```python
from build123d import *

# Parameters (mm, degrees)
SKETCH1_R               = 10
BOSS_EXTRUDE1_DEPTH     = 2
CUT_EXTRUDE1_REACH      = 16.283
CUT_EXTRUDE1_END_RADIUS = 10
SKETCH2_R               = 1.5
CUT_EXTRUDE1_DRAFT      = 2
CIRPATTERN1_COUNT       = 3


with BuildPart() as part:
    # Sketch1 → Boss-Extrude1 (new, symmetric)
    with BuildSketch(Plane(origin=(0, 0, 0), x_dir=(1, 0, 0), z_dir=(0, 1, 0))):
        with Locations(Location((0, 0, 0), (0, 0, 270))):
            Circle(SKETCH1_R)
        Polygon((0, 3.868246804), (-3.35, 1.934123402), (-3.35, -1.934123402), (0, -3.868246804), (3.35, -1.934123402), (3.35, 1.934123402), align=None, mode=Mode.SUBTRACT)
    extrude(amount=BOSS_EXTRUDE1_DEPTH, both=True)

    # Cut-Extrude1: up to this cylinder (the profile starts inside it)
    cut_extrude1_end = Plane(origin=(0, 0, 0), z_dir=(0, -1, 0)) * Cylinder(CUT_EXTRUDE1_END_RADIUS, 53.566, mode=Mode.PRIVATE)



with BuildPart() as cut_extrude1_long_prism_1:
    # Sketch2 → Cut-Extrude1 (the long prism of profile 1, to be tilted and cut off)
    with BuildSketch(Plane.XY):
        Circle(SKETCH2_R)
    extrude(amount=CUT_EXTRUDE1_REACH)
    cut_extrude1_tool1_sides = [cut_extrude1_long_prism_1.faces().sort_by_distance(p)[0] for p in [
        (-1.5, 0, 8.1415),
    ]]
    draft(cut_extrude1_tool1_sides, Plane.XY, CUT_EXTRUDE1_DRAFT)  # the draft: side faces tilted about the start plane


with BuildPart() as part_1:
    add(part.part)
    cut_extrude1_tool1 = cut_extrude1_long_prism_1.part & cut_extrude1_end
    cut_extrude1 = cut_extrude1_tool1.solids().sort_by_distance((0, 0, 0))[0]
    add(cut_extrude1, mode=Mode.SUBTRACT)

    # CirPattern1: Cut-Extrude1 ×3 about axis
    cirpattern1_axis = Axis((0, 2, 0), (0, -1, 0))
    for i in range(1, CIRPATTERN1_COUNT):
        add(cut_extrude1.rotate(cirpattern1_axis, i * 360 / CIRPATTERN1_COUNT), mode=Mode.SUBTRACT)


solid = part_1.part
```
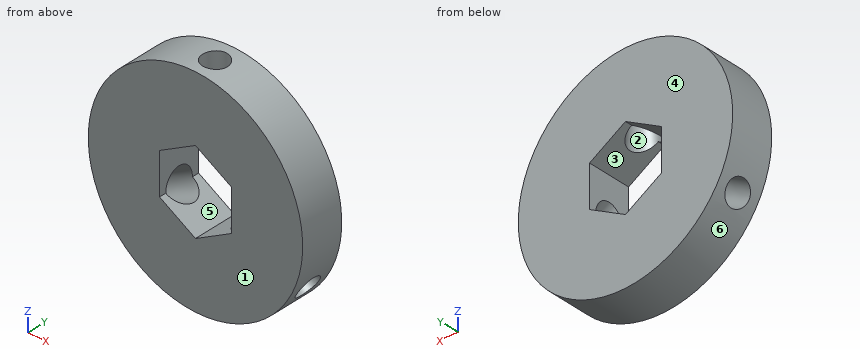
Geometry: final body of the model. Coordinates: model frame, mm. Face numbers are marked on the shaded views. A direction names the side the tool comes from. Give positions to 0.01 mm unless a question says otherwise; leave off trailing zeros. Order: outer loops, then holes, each group sorted by start corner. A loop starts at its lowest first (then second) coordinate and runs counter-clockwise, first axis right, second up. Notation, with made-up numbers: M -2,-30.5 L 15,-30.5 A12 cw 15,-15.5 Z; hole C -33.75,39 d9. An arc over 180 degrees is marked long. Answer as CSV lines item,"result". Start each with the question number.
1) First-contact query: P1, Ø1.5, axis at y = 1.5, z = 6, coming from the +X side; P2, Ø1, axis at x = 2, y = -1.5, coming from the -Z side; P3, Ø1.5, axis at x = -2.5, y = -1.5, coming from the +Z side. Flat tips, straight axial feed; report the tip coordinate or a pass-through.
2) Cut plane B-B (y = 0). Output: boundary loops of the cut face in (x, z), then the cut area to 3 significant figures.
3) Line query: line 1 (X direction, y = 1.65, z = 0); line 2 (X direction, y = 1.45, z = 2); line 3 (Y direction, x = -1, z = 7.5). Output: solid intervals per line, ascending. Write a range as from..to.
4) Mould query, pull axis X, two halves, no side actions, for the marked faces 4, 5 and 6. Classes: +X half, -X half, draft (parallel to the pull), parting line (faces both ways), or undercut.
5) Cut plane A-A (z = 0). Output: boundary loops of the cut face in (x, y), then the cut area to 3 significant figures.
6) Set-up query: the marked faces 1, 2 and 3. Return all of +Z, -Z, +X, -X, +Y, -Y with unobstructed straight access to the full face (end or side cutting, diameter ignored); none if empty.
Findings below:
1,P1,"stops at x = 8.51"
1,P2,"stops at z = -9.89"
1,P3,"stops at z = 9.85"
2,outline,"M -9.18,-3.97 L -3.35,-0.33 L -3.35,1.93 L -1.39,3.06 L -1.15,9.93 A10 ccw Z; M -8.03,-5.97 A10 ccw 8.03,-5.97 L 1.96,-2.74 L 0,-3.87 L -1.96,-2.74 Z; M 1.15,9.93 L 1.39,3.06 L 3.35,1.93 L 3.35,-0.33 L 9.18,-3.97 A10 ccw Z"
2,area,"226 mm²"
3,line 1,"x = -10..-3.35, 3.35..10"
3,line 2,"x = -9.8..-3.24, 3.24..9.8"
3,line 3,"y = -2..-0.73, 0.73..2"
4,face 4,"draft"
4,face 5,"undercut"
4,face 6,"parting line"
5,outline,"M -10,-2 L -3.35,-2 L -3.35,2 L -10,2 Z; M 3.35,-2 L 10,-2 L 10,2 L 3.35,2 Z"
5,area,"53.2 mm²"
6,face 1,"+Z, -Z, +X, -X, -Y"
6,face 2,"none"
6,face 3,"+Y, -Y"
